```python
from build123d import *

# Parameters (mm, degrees)
SKETCH1_W           = 105
SKETCH1_H           = 65
BOSS_EXTRUDE1_DEPTH = 10
SKETCH2_W           = 61
SKETCH2_H           = 31
CUT_EXTRUDE1_DEPTH  = 63.549980016
SKETCH4_R           = 3.125
SKETCH4_W           = 2.5
SKETCH4_H           = 6.35
CUT_EXTRUDE3_DEPTH  = 63.549980016
BOSS_EXTRUDE2_DEPTH = 10
SKETCH6_R           = 3.075
CUT_EXTRUDE4_DEPTH  = 85.949986617
FILLET1_R           = 4
FILLET2_R           = 0.5


with BuildPart() as part:
    # Sketch1 → Boss-Extrude1 (new body)
    with BuildSketch(Plane(origin=(0, 0, 0), x_dir=(1, 0, 0), z_dir=(0, 1, 0))):
        Rectangle(SKETCH1_W, SKETCH1_H)
    extrude(amount=BOSS_EXTRUDE1_DEPTH)

    # Sketch2 → Cut-Extrude1 (cut, through all)
    with BuildSketch(Plane(origin=(0, 10, 0), x_dir=(1, 0, 0), z_dir=(0, 1, 0))):
        with Locations((0, 8)):
            Rectangle(SKETCH2_W, SKETCH2_H)
    extrude(amount=-CUT_EXTRUDE1_DEPTH, mode=Mode.SUBTRACT)

    # Sketch4 → Cut-Extrude3 (cut, through all)
    with BuildSketch(Plane(origin=(0, 10, 0), x_dir=(1, 0, 0), z_dir=(0, 1, 0))):
        with Locations(Location((-46.5, 8.5, 0), (0, 0, 270))):
            Circle(SKETCH4_R)
        with Locations((-34.5, 8.5)):
            Rectangle(SKETCH4_W, SKETCH4_H)
    cut_extrude3 = extrude(amount=-CUT_EXTRUDE3_DEPTH, mode=Mode.SUBTRACT)

    # Sketch5 → Boss-Extrude2 (add)
    with BuildSketch(Plane(origin=(0, 0, 0), x_dir=(1, 0, 0), z_dir=(0, 1, 0))):
        with BuildLine():
            Line((0, -32.5), (-52.5, -19.039128985))
            Line((-52.5, -19.039128985), (-56.408079011, -62.726619731))
            add(Edge.make_bspline(
                [(0, -32.5), (-47.244656315, -32.5), (-56.408079011, -62.726619731)],
                knots=[4.71238898, 4.71238898, 4.71238898, 6.087991355, 6.087991355, 6.087991355], degree=2, weights=[1, 0.772643775, 1]))
        make_face()
    boss_extrude2 = extrude(amount=BOSS_EXTRUDE2_DEPTH)

    # Sketch6 → Cut-Extrude4 (cut, through all)
    with BuildSketch(Plane(origin=(0, 10, 0), x_dir=(1, 0, 0), z_dir=(0, 1, 0))):
        with Locations(Location((-43.347709835, 23.330814615, 0), (0, 0, 270))):
            Circle(SKETCH6_R)
    cut_extrude4 = extrude(amount=-CUT_EXTRUDE4_DEPTH, mode=Mode.SUBTRACT)

    # Mirror1: Cut-Extrude3, Boss-Extrude2, Cut-Extrude4 across plane
    add(cut_extrude3.mirror(Plane(origin=(0, 0, 0), x_dir=(0, 0, 1), z_dir=(1, 0, 0))), mode=Mode.SUBTRACT)
    add(boss_extrude2.mirror(Plane(origin=(0, 0, 0), x_dir=(0, 0, 1), z_dir=(1, 0, 0))))
    add(cut_extrude4.mirror(Plane(origin=(0, 0, 0), x_dir=(0, 0, 1), z_dir=(1, 0, 0))), mode=Mode.SUBTRACT)

    # Fillet1
    # the kernel refuses this fillet: 4 mm, written as the material it adds along each edge
    with BuildSketch(Plane(origin=(-52.5, 0, 19.039128985), x_dir=(0, 0, -1), z_dir=(0, 1, 0))) as fillet1_piece_1:
        with BuildLine():
            CenterArc((FILLET1_R * 0.0446385419256, FILLET1_R), FILLET1_R, 264.888193347, 5.111806653)
            Line((-FILLET1_R * 0.0444610022252, FILLET1_R * 0.00397727373713), (0, 0))
            Line((0, 0), (FILLET1_R * 0.0446385419256, 0))
        make_face()
    extrude(amount=10)
    with BuildSketch(Plane(origin=(52.5, 0, 19.039128985), x_dir=(0, 0, -1), z_dir=(0, 1, 0))) as fillet1_piece_2:
        with BuildLine():
            CenterArc((FILLET1_R * 0.0446385419256, -FILLET1_R), FILLET1_R, 90, 5.111806653)
            Line((-FILLET1_R * 0.0444610022252, -FILLET1_R * 0.00397727373713), (0, 0))
            Line((0, 0), (FILLET1_R * 0.0446385419256, 0))
        make_face()
    extrude(amount=10)
    # the kernel refuses this fillet: 4 mm, written as the material it takes off along each edge
    with BuildSketch(Plane(origin=(-52.5, -10, -32.5), x_dir=(0, 0, 1), z_dir=(0, 1, 0)), Plane(origin=(52.5, -10, -32.5), x_dir=(-1, 0, 0), z_dir=(0, 1, 0))) as fillet1_2_piece_1:
        with BuildLine():
            CenterArc((FILLET1_R, FILLET1_R), FILLET1_R, 180, 90)
            Line((0, FILLET1_R), (0, 0))
            Line((0, 0), (FILLET1_R, 0))
        make_face()
    extrude(amount=30, mode=Mode.SUBTRACT)

    # Fillet2
    fillet2_edges = [part.edges().sort_by_distance(p)[0] for p in [
        (56.408079011, 5, 62.726619731),
        (-56.408079011, 5, 62.726619731),
    ]]
    fillet(fillet2_edges, radius=FILLET2_R)


solid = part.part
```
The listing builds one solid part. Answer for the finished solid, in the listing's coordinates (mm). A direction names the side the tool comes from. Give positions to 0.01 mm unless a question says otherwise; leave off trailing zeros. Order: outer loops, then holes, each group sorted by start corner. A loop starts at its lowest first (then second) coordinate and runs counter-clockwise, first axis right, second up. Notation, with made-up numbers: (-10, -7) - (13, -7) arc R34 cw to (13, 27) - close; hole circle Ø4 at (8.25, 79.5). An arc over 180 degrees is marked (long way). Use one line per item in the form item = value. Start each with the question number.
(1) For faces 1 (the flat face through (-52.5, 5, -4)), 2 (the flat face through (30.5, 5, -8)), 3 (the flat face through (52.5, 5, -4)), 4 (the flat face through (-1, 5, -32.5)), determine the directions among +Z, -Z, +X, -X, +Y, -Y from which every point of the face is accessible in a straight line to the end or side of a thin tool.
(2) A cutting plane is placed at B-B, the plane z = -8.5. Write down the section's boundary in (x, y) (3 decimals), then the cut area to 3 significant figures.
(3) A cutting plane is placed at A-A, the plane z = 5.5. Write down the section's boundary in (x, y), then the cut area to 3 significant figures.
(4) The mould has two halves that part along X. Classify faces 5 (the cylindrical face through (-51.297, 4.93, -31.359)), 6 (the flat face through (-1, 10, 13)), 7 (the cylindrical face through (43.4, 5.1, -8.9)), 8 (the flat face through (35, 5, -11.675)): released by +X, released by -X, zero draft, split by the parting line, or undercut.
(5) Flat-ended cylindrical pins translate along their axes: pin 1 Ø5 at (y, z) = (6, -9.5) entering from +X; pin 2 Ø10 at (x, z) = (46.5, -8.5) entering from +Y; pin 3 Ø1 at (y, z) = (7.5, 45) entering from +X; pin 4 Ø1.2 at (x, y) = (-34, 7.5) entering from +Z. Find the tip coordinate at first contact, or state that the pin passes through.
(6) A cutting plane is placed at C-C, the plane y = 7.75. State how many separate pieces and enclosed holes the cut face has, then the cut area to 3 significant figures.
(7) Consider line 1 (X direction, y = 4.5, z = -8.5) (3 decimals); line 2 (X direction, y = 7, z = -17); line 3 (Z direction, x = 11.5, y = 5.5). Determine where each line is inside the solid, lowest interval first. Write a range as from..to.
Ans:
q1.face_1 = -Z, -X, +Y, -Y
q1.face_2 = +Y, -Y
q1.face_3 = -Z, +X, +Y, -Y
q1.face_4 = -Z, +X, -X, +Y, -Y
q2.outline = (-52.5, 0) - (-49.625, 0) - (-49.625, 10) - (-52.5, 10) - close; (-43.375, 0) - (-35.75, 0) - (-35.75, 10) - (-43.375, 10) - close; (-33.25, 0) - (-30.5, 0) - (-30.5, 10) - (-33.25, 10) - close; (30.5, 0) - (33.25, 0) - (33.25, 10) - (30.5, 10) - close; (35.75, 0) - (43.375, 0) - (43.375, 10) - (35.75, 10) - close; (49.625, 0) - (52.5, 0) - (52.5, 10) - (49.625, 10) - close
q2.area = 265 mm^2
q3.outline = (-52.5, 0) - (-30.5, 0) - (-30.5, 10) - (-52.5, 10) - close; (30.5, 0) - (52.5, 0) - (52.5, 10) - (30.5, 10) - close
q3.area = 440 mm^2
q4.face_5 = released by -X
q4.face_6 = zero draft
q4.face_7 = undercut
q4.face_8 = undercut
q5.pin_1 = 52.5
q5.pin_2 = 10
q5.pin_3 = 54.87
q5.pin_4 = 40.05
q6.separate_pieces = 1
q6.enclosed_holes = 7
q6.area = 5,560 mm^2
q7.line_1 = -52.5..-49.625, -43.375..-35.75, -33.25..-30.5, 30.5..33.25, 35.75..43.375, 49.625..52.5
q7.line_2 = -52.5..-30.5, 30.5..52.5
q7.line_3 = -32.5..-23.5, 7.5..33.26
